```python
from build123d import *

# Parameters (mm, degrees)
BOSS_EXTRUDE2_DEPTH = 20
SKETCH2_W           = 10
SKETCH2_H           = 14
SKETCH2_R           = 2.75
SKETCH2_R_2         = 2.25
BOSS_EXTRUDE3_DEPTH = 4
SKETCH6_R           = 4
CUT_EXTRUDE1_DEPTH  = 2


with BuildPart() as part:
    # Sketch1 → Boss-Extrude2 (new, symmetric)
    with BuildSketch(Plane(origin=(0, 0, 0), x_dir=(0, 0, -1), z_dir=(1, 0, 0))):
        with BuildLine():
            Line((-13.919410907, 1.5), (-9.886859967, 1.5))
            ThreePointArc((-9.886859967, 1.5), (0, 10), (9.886859967, 1.5))
            Line((9.886859967, 1.5), (13.919410907, 1.5))
            ThreePointArc((13.919410907, 1.5), (0, 14), (-13.919410907, 1.5))
        make_face()
    extrude(amount=BOSS_EXTRUDE2_DEPTH, both=True)

    # Sketch2 → Boss-Extrude3 (add)
    # profile 1 of 4: a face of its own
    with BuildSketch(Plane.XZ.offset(-1.5)):
        with Locations((-15, -16.886859967)):
            Rectangle(SKETCH2_W, SKETCH2_H)
        with Locations(Location((-15, -18.903135437, 0), (0, 0, 270))):
            Circle(SKETCH2_R, mode=Mode.SUBTRACT)
    # profile 2 of 4: a face of its own
    with BuildSketch(Plane.XZ.offset(-1.5)):
        with Locations((15, -16.886859967)):
            Rectangle(SKETCH2_W, SKETCH2_H)
        with Locations(Location((15, -18.903135437, 0), (0, 0, 270))):
            Circle(SKETCH2_R_2, mode=Mode.SUBTRACT)
    # profile 3 of 4: a face of its own
    with BuildSketch(Plane.XZ.offset(-1.5)):
        with Locations((-15, 16.886859967)):
            Rectangle(SKETCH2_W, SKETCH2_H)
        with Locations(Location((-15, 18.903135437, 0), (0, 0, 270))):
            Circle(SKETCH2_R_2, mode=Mode.SUBTRACT)
    # profile 4 of 4: a face of its own
    with BuildSketch(Plane.XZ.offset(-1.5)):
        with Locations((15, 16.886859967)):
            Rectangle(SKETCH2_W, SKETCH2_H)
        with Locations(Location((15, 18.903135437, 0), (0, 0, 270))):
            Circle(SKETCH2_R, mode=Mode.SUBTRACT)
    extrude(amount=-BOSS_EXTRUDE3_DEPTH)

    # Sketch6 → Cut-Extrude1 (cut)
    with BuildSketch(Plane.XZ.offset(-1.5)):
        with Locations(Location((-15, 18.903135437, 0), (0, 0, 270))):
            Circle(SKETCH6_R)
        with Locations(Location((15, -18.903135437, 0), (0, 0, 270))):
            Circle(SKETCH6_R)
    extrude(amount=-CUT_EXTRUDE1_DEPTH, mode=Mode.SUBTRACT)


solid = part.part
```
Model file for the job. Use its own axes, mm. A direction names the side the tool comes from. Give positions to 0.01 mm unless a question says otherwise; leave off trailing zeros. Order: outer loops, then holes, each group sorted by start corner. A loop starts at its lowest first (then second) coordinate and runs counter-clockwise, first axis right, second up.
1) Pin check, flat tips, straight feed: pin 1 (6 mm diameter, centred on x = 15, z = -18.9, fed in from -Y); pin 2 (5 mm diameter, centred on x = -4.5, z = -12.5, fed in from +Y); pin 3 (9 mm diameter, centred on x = -15, z = 18.9, fed in from +Y). Stop position of each tip, or through.
2) Mould opens along X. For faces 4 (the flat face through (10, 3, -18)), 5 (the flat face through (-15, 3, -23.887)) say: +X half, -X half, draft (parallel to the pull), parting line (faces both ways), or undercut.
3) Wall check: probe 1 along X at (y, z) = (4, -19); probe 2 along X at (y, z) = (2, 16); probe 3 along X at (y, z) = (4.5, -17.5). Give the ranges that are in metal, low to high.
4) Saw through at A-A, the plane x = 15. Write the cut outline in (y, z).
5) Saw through at C-C, the plane y = 7.5. Write the cut outline in (x, z).
6) 3-axis set-ups, long thin cutter, end or side, ignore diameter. For faces 1 (the cylindrical face through (0, 14, 0)), 2 (the flat face through (13, 3.5, -21)), 3 (the flat face through (-15, 5.5, 16)): which of +Z, -Z, +X, -X, +Y, -Y reach the whole face in a straight line?
7) Saw through at D-D, the plane x = -3. Write the cut outline in (y, z).
8) Saw through at B-B, the plane y = 4.75. Write the cut outline in (x, z).
Computed:
1. pin 1: stops at y = 3.5
1. pin 2: stops at y = 9.8
1. pin 3: stops at y = 5.5
2. face 4: undercut
2. face 5: draft
3. probe 1: x = -20 to -17.75, -12.25 to -10, 10 to 12.75, 17.25 to 20
3. probe 2: x = -20 to -17.75, -12.25 to -10, 10 to 20
3. probe 3: x = -20 to -17.37, -12.63 to -10, 10 to 13.24, 16.76 to 20
4. outline: (1.5, -23.89) - (5.5, -23.89) - (5.5, -21.15) - (3.5, -21.15) - (3.5, -22.9) - (1.5, -22.9) - close; (1.5, -14.9) - (3.5, -14.9) - (3.5, -16.65) - (5.5, -16.65) - (5.5, -12.87) arc R14 ccw to (5.5, 12.87) - (5.5, 16.15) - (1.5, 16.15) - (1.5, 9.89) arc R10 cw to (1.5, -9.89) - close; (1.5, 21.65) - (5.5, 21.65) - (5.5, 23.89) - (1.5, 23.89) - close
5. outline: (-20, -11.82) - (20, -11.82) - (20, -6.61) - (-20, -6.61) - close; (-20, 6.61) - (20, 6.61) - (20, 11.82) - (-20, 11.82) - close
6. face 1: +Y
6. face 2: -Y
6. face 3: +Z, +X, -X, +Y
7. outline: (1.5, -13.92) arc R14 ccw to (1.5, 13.92) - (1.5, 9.89) arc R10 cw to (1.5, -9.89) - close
8. outline: (-20, -23.89) - (-10, -23.89) - (-10, -13.17) - (10, -13.17) - (10, -23.89) - (20, -23.89) - (20, -8.8) - (-20, -8.8) - close; (-20, 8.8) - (20, 8.8) - (20, 23.89) - (10, 23.89) - (10, 13.17) - (-10, 13.17) - (-10, 23.89) - (-20, 23.89) - close; hole circle Ø5.5 at (-15, -18.9); hole circle Ø4.5 at (-15, 18.9); hole circle Ø5.5 at (15, 18.9); hole circle Ø4.5 at (15, -18.9)
